Work out the finished part from the listing and answer in its coordinate system (mm). A direction names the side the tool comes from. Give positions to 0.01 mm unless a question says otherwise; leave off trailing zeros. Loops run counter-clockwise (first coordinate to the right, second up) from the corner with the lowest first, then second, coordinate; pieces in that order, holes last. Notation, with made-up numbers: (-19.75, -15.5) -> (8.25, -15.5) arc R23 cw to (8.25, -0.5) -> close; hole circle Ø10 at (28, 52). An arc over 180 degrees is marked (long way). Answer as CSV lines item,"result". Start each with the question number.
1. A tool of negligible diameter and unlimited length cuts with its end or side. For faces 1 (the face through (-0.671, 1.875, -3.02)), 2 (the face through (0, 12, -2)), from which of +Z, -Z, +X, -X, +Y, -Y can it reach the whole face along a straight path? Write none if from no direction.
2. Find the intervals of material crossed by line 1 along Z through (x, y) = (0, 8.5); line 2 along Z through (x, y) = (0, 3.25); line 3 along Y through (x, z) = (-3.25, 0.5), in increasing order.
3. Flat-ended cylindrical pins translate along their axes: pin 1 Ø3 at (x, z) = (0, 0) entering from -Y; pin 2 Ø1 at (y, z) = (6, 3.5) entering from -X; pin 3 Ø4 at (y, z) = (5.5, 0) entering from +X; pin 4 Ø2 at (x, y) = (-0.5, 6.5) entering from -Z. Find the tip coordinate at first contact, or state that the pin passes through.
4. Determine the mould class of faces 3 (the face through (-0.27, 5.92, -1.22)), 4 (the face through (1, 0, -1)), 5 (the face through (3.233, 8.238, 1.341)) for opening direction Z: +Z half, -Z half, draft (parallel to the pull), parting line (faces both ways), or undercut.
5. Find section B-B, the plane z = 0. Give the vertices of the cut face in (x, y).
6. Find section A-A, the plane x = 0. Give the vertices of the cut face in (y, z).
7. Find section C-C, the plane y = 10.5. Give the vertices of the cut face in (x, z), and give its area (3 significant figures).
Autodesk Inventor part; units mm, degrees
ref_plane "PAD_DUMMY_XY" through (0, 0, 0) normal (0, -1, 0) x (1, 0, 0)
ref_plane "PAD_DUMMY_YZ" through (0, 0, 0) normal (1, 0, 0) x (0, 0, 1)
ref_plane "PAD_DUMMY_ZX" through (0, 0, 0) normal (0, 0, 1) x (0, -1, 0)
sketch "Sketch_3" plane through (0, 0, 0) normal (0, 0, 1) x (1, 0, 0)
  line L0 (0, 0) -> (0, 12)
  line L1 (1.25, 12) -> (1.25, 0)
  line L2 (1.25, 0) -> (4.5, 0)
  line L3 (4.5, 0) -> (3, 2)
  line L4 (3, 2) -> (3, 3.5)
  line L5 (3, 3.5) -> (3.5, 4.37)
  line L6 (3.5, 4.37) -> (3.5, 12)
  line L7 (3.5, 12) -> (1.25, 12)
revolve "Revolution1" add sketch "Sketch_3" angle 360 about axis through (0, 0, 0) along (0, -1, 0)
ref_plane "PAD_DUMMY_XY" through (0, 0, 0) normal (0, -1, 0) x (1, 0, 0)
ref_plane "PAD_DUMMY_YZ" through (0, 0, 0) normal (1, 0, 0) x (0, 0, 1)
ref_plane "PAD_DUMMY_ZX" through (0, 0, 0) normal (0, 0, 1) x (0, -1, 0)
ref_plane "pad_a_XY" through (0, 12, 0) normal (0, 1, 0) x (1, 0, 0)
ref_plane "pad_a_YZ" through (0, 12, 0) normal (1, 0, 0) x (0, 0, -1)
ref_plane "pad_a_ZX" through (0, 12, 0) normal (0, 0, -1) x (0, 1, 0)
properties part number "ZP08U_T_B"
Resolved:
1,face 1,"none"
1,face 2,"+Z, -Z, +X, -X, +Y"
2,line 1,"z = -3.5 to -1.25, 1.25 to 3.5"
2,line 2,"z = -3 to -1.25, 1.25 to 3"
2,line 3,"y = 0 to 1.62, 4 to 12"
3,pin 1,"stops at y = 0"
3,pin 2,"stops at x = -1.8"
3,pin 3,"stops at x = 3.5"
3,pin 4,"stops at z = -3.5"
4,face 3,"undercut"
4,face 4,"draft"
4,face 5,"parting line"
5,outline,"(-4.5, 0) -> (-1.25, 0) -> (-1.25, 12) -> (-3.5, 12) -> (-3.5, 4.37) -> (-3, 3.5) -> (-3, 2) -> close; (1.25, 0) -> (4.5, 0) -> (3, 2) -> (3, 3.5) -> (3.5, 4.37) -> (3.5, 12) -> (1.25, 12) -> close"
6,outline,"(0, -4.5) -> (2, -3) -> (3.5, -3) -> (4.37, -3.5) -> (12, -3.5) -> (12, -1.25) -> (0, -1.25) -> close; (0, 1.25) -> (12, 1.25) -> (12, 3.5) -> (4.37, 3.5) -> (3.5, 3) -> (2, 3) -> (0, 4.5) -> close"
7,outline,"circle Ø7 at (0, 0); hole circle Ø2.5 at (0, 0)"
7,area,"33.6 mm^2"
